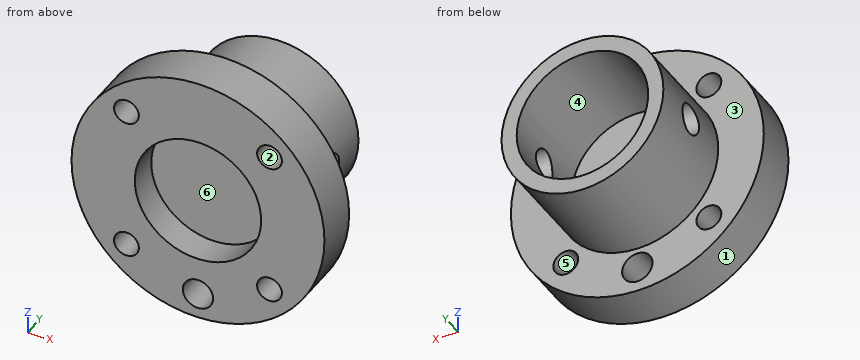
Autodesk Inventor part; units mm, degrees
ref_plane "Work Plane1" through (16, 9, 0) normal (1, 0, 0) x (0, 1, 0)
ref_plane "XZ Plane" through (0, 0, 0) normal (0, 1, 0) x (-1, 0, 0)
ref_plane "XY Plane" through (0, 0, 0) normal (0, 0, 1) x (1, 0, 0)
sketch "Sketch1" plane through (0, 0, 0) normal (0, 1, 0) x (-1, 0, 0)
  circle A0 centre (0, 0) radius 25
  dimension "d0" = 50
extrude "Extrusion1" add sketch "Sketch1" along normal blind 9
sketch "Sketch2" plane through (0, 0, 0) normal (0, -1, 0) x (1, 0, 0)
  circle A0 centre (0, 0) radius 12.5
  dimension "d3" = 25
extrude "Extrusion2" cut sketch "Sketch2" against normal blind 6
sketch "Sketch3" plane through (0, 9, 0) normal (0, 1, 0) x (1, 0, 0)
  circle A0 centre (0, 0) radius 20
  line L0 (0, 35) -> (0, -35)
  line L1 (0, 0) -> (14.1421, 14.1421)
  line L2 (-35, 0) -> (35, 0)
  point P0 (0, 20)
  dimension "d6" = 40
  dimension "d15" = 45
hole "Hole1" at (0, 9, -20) direction (0, -1, 0) diameter 6 end through all
hole "Hole2" at (14.1421, 9, -14.1421) direction (0, -1, 0) diameter 4.917 end through all
pattern_circular "Circular Pattern1" count 4 over 360 about axis through (0, 0, 0) along (0, 1, 0) of "Hole2"
sketch "Sketch8" plane through (0, 9, 0) normal (0, 1, 0) x (1, 0, 0)
  circle A0 centre (0, 0) radius 16
  dimension "d49" = 32
extrude "Extrusion5" add sketch "Sketch8" along normal blind 20
ref_plane "Work Plane1" through (16, 9, 0) normal (1, 0, 0) x (0, 1, 0)
sketch "Sketch15" plane through (16, 9, 0) normal (1, 0, 0) x (0, 1, 0)
  line L0 (0, -16) -> (20, -16)
  line L1 (20, -16) -> (20, 16)
  line L2 (-14.8, 0) -> (25.8, 0)
  point P0 (-9, 0)
  point P1 (10, 0)
  dimension "d60" = 10
  dimension "d61" = 20
hole "Hole4" at (16, 19, 0) direction (-1, 0, 0) diameter 6 end through all
sketch "Sketch16" plane through (0, 29, 0) normal (0, 1, 0) x (1, 0, 0)
  circle A0 centre (0, 0) radius 13
  circle A1 centre (0, 0) radius 16
  dimension "d70" = 3
extrude "Extrusion7" cut sketch "Sketch16" against normal up to surface (20 mm away) contours A0
properties part number "Brida para herramienta"
Geometry check sheet. Reference: the model listing, model coordinates, mm. Face numbers are marked on the shaded views. A direction names the side the tool comes from. Round coordinates to 2 decimals unless told otherwise and drop trailing zeros. Loops run counter-clockwise (first coordinate to the right, second up) from the corner with the lowest first, then second, coordinate; pieces in that order, holes last. Notation, with made-up numbers: (60.5, 53.25) - (116.5, 53.25) arc R5 ccw to (116.5, 59.25) - close; hole circle Ø1 at (56, 22.5). An arc over 180 degrees is marked (long way). Write item = value, one per line. Start each with the question number.
1. Section check C-C on z = -20. Enter the section's corners in (x, y).
2. Section check D-D on y = 19. Enter the section's corners in (x, z), then the cut area to 3 significant figures.
3. Mould release check, pull along X, two halves, no side actions. Record for the marked faces 1, 2 and 3: released by +X, released by -X, zero draft, split by the parting line, or undercut.
4. Thickness scan on line 1 (Y direction, x = -14.25, z = 0); line 2 (X direction, y = 13.5, z = 0.5); line 3 (X direction, y = 20.5, z = -3.5). Record the ranges inside material, lowest first.
5. Section check B-B on x = 0. Enter the section's corners in (y, z), then the cut area to 3 significant figures.
6. Depth check by flat-ended pin: pin 1 (3 mm diameter, centred on x = 14.14, z = 14.14, fed in from -Y); pin 2 (1 mm diameter, centred on x = -9.5, z = -5.5, fed in from +Y); pin 3 (12.5 mm diameter, centred on x = 2.5, z = 5.5, fed in from -Y); pin 4 (5 mm diameter, centred on y = 23, z = -4, fed in from -X). Enter the tip coordinate at first touch or a pass-through.
7. Set-up check for the marked faces 4, 5 and 6: record each of +Z, -Z, +X, -X, +Y, -Y from which the full face is reachable in a straight line by a thin tool's end or side.
8. Section check A-A on z = 0. Enter the section's corners in (x, y).
Working result:
q1.outline = (-15, 0) - (-3, 0) - (-3, 9) - (-15, 9) - close; (3, 0) - (15, 0) - (15, 9) - (3, 9) - close
q2.outline = (-15.72, -3) arc R16 ccw to (15.72, -3) - (12.65, -3) arc R13 cw to (-12.65, -3) - close; (-15.72, 3) - (-12.65, 3) arc R13 cw to (12.65, 3) - (15.72, 3) arc R16 ccw to start
q2.area = 237 mm^2
q3.face_1 = split by the parting line
q3.face_2 = undercut
q3.face_3 = zero draft
q4.line_1 = 0 to 16, 22 to 29
q4.line_2 = -15.99 to -12.99, 12.99 to 15.99
q4.line_3 = -15.61 to -12.52, 12.52 to 15.61
q5.outline = (0, -25) - (9, -25) - (9, -23) - (0, -23) - close; (0, -17) - (9, -17) - (9, -16) - (29, -16) - (29, -13) - (9, -13) - (9, 13) - (29, 13) - (29, 16) - (9, 16) - (9, 25) - (0, 25) - (0, 12.5) - (6, 12.5) - (6, -12.5) - (0, -12.5) - close
q5.area = 366 mm^2
q6.pin_1 = through
q6.pin_2 = 9
q6.pin_3 = 6
q6.pin_4 = -15.93
q7.face_4 = +Y
q7.face_5 = +Y, -Y
q7.face_6 = -Y
q8.outline = (-25, 0) - (-12.5, 0) - (-12.5, 6) - (12.5, 6) - (12.5, 0) - (25, 0) - (25, 9) - (16, 9) - (16, 16) - (13, 16) - (13, 9) - (-13, 9) - (-13, 16) - (-16, 16) - (-16, 9) - (-25, 9) - close; (-16, 22) - (-13, 22) - (-13, 29) - (-16, 29) - close; (13, 22) - (16, 22) - (16, 29) - (13, 29) - close
